Geometry check sheet. Reference: the model listing, model coordinates, mm. A direction names the side the tool comes from. Coordinates: 2 decimals unless noted, no trailing zeros. Loops run counter-clockwise (first coordinate to the right, second up) from the corner with the lowest first, then second, coordinate; pieces in that order, holes last.
from build123d import *

# Parameters (mm, degrees)
F0_W     = 33
F0_H     = 14
F1_DEPTH = 10
F2_W     = 33
F2_H     = 10.2
F3_DEPTH = 2
F4_D     = 3
F4_DEPTH = 20.5
F4_TIP   = 0.9012909285
F6_D     = 2.3
F6_DEPTH = 20.5
F6_TIP   = 0.6909897119


with BuildPart() as f1:
    # F0 (on Top) → F1 (new body)
    with BuildSketch(Plane.XY):
        Rectangle(F0_W, F0_H)
    extrude(amount=F1_DEPTH)

    # F2 (on face) → F3 (cut)
    with BuildSketch(Plane.XY.offset(10)):
        Rectangle(F2_W, F2_H)
    extrude(amount=-F3_DEPTH, mode=Mode.SUBTRACT)

    # F4
    with Locations(Plane(origin=(0, 0, 0), x_dir=(1, 0, 0), z_dir=(0, 0, -1))):
        with Locations((-12, 0)):
            Hole(F4_D / 2, depth=F4_DEPTH)
            with Locations((0, 0, -(F4_DEPTH + F4_TIP / 2))):  # 118° drill point
                Cone(0, F4_D / 2, F4_TIP, mode=Mode.SUBTRACT)

    # F6
    with Locations(Plane.YZ.offset(16.5)):
        with Locations((0, 4)):
            Hole(F6_D / 2, depth=F6_DEPTH)
            with Locations((0, 0, -(F6_DEPTH + F6_TIP / 2))):  # 118° drill point
                Cone(0, F6_D / 2, F6_TIP, mode=Mode.SUBTRACT)


solid = f1.part
1) Access from +Z, -Z, +X, -X, +Y, -Y to the whole of each face (thin tool, end or side, straight path). Record for faces 1 (the flat face through (0, 0, 8)), 2 (the cylindrical face through (6.11, 0.15, 5.14)), 3 (the flat face through (0, -6, 10)).
Data:
face 1: +Z, +X, -X
face 2: +X
face 3: +Z, +X, -X, +Y, -Y
2) Section check A-A on x = -12. Record the cut outline in (y, z).
Data:
outline: (-7, 0) - (-1.5, 0) - (-1.5, 8) - (-5.1, 8) - (-5.1, 10) - (-7, 10) - close; (1.5, 0) - (7, 0) - (7, 10) - (5.1, 10) - (5.1, 8) - (1.5, 8) - close
3) Section check D-D on x = -8. Record the cut outline in (y, z).
Data:
outline: (-7, 0) - (7, 0) - (7, 10) - (5.1, 10) - (5.1, 8) - (-5.1, 8) - (-5.1, 10) - (-7, 10) - close
4) Section check C-C on x = 2. Record the cut outline in (y, z).
Data:
outline: (-7, 0) - (7, 0) - (7, 10) - (5.1, 10) - (5.1, 8) - (-5.1, 8) - (-5.1, 10) - (-7, 10) - close; hole circle Ø2.3 at (0, 4)
5) Depth check by flat-ended pin: pin 1 (2 mm diameter, centred on y = 0, z = 4, fed in from +X); pin 2 (4 mm diameter, centred on x = -12.5, y = -3, fed in from +Z); pin 3 (2.5 mm diameter, centred on x = -12, y = 0, fed in from +Z). Enter the tip coordinate at first touch or a pass-through.
Data:
pin 1: stops at x = -4.09
pin 2: stops at z = 8
pin 3: passes through
6) Section check B-B on z = 8.75. Record the cut outline in (x, y).
Data:
outline: (-16.5, -7) - (16.5, -7) - (16.5, -5.1) - (-16.5, -5.1) - close; (-16.5, 5.1) - (16.5, 5.1) - (16.5, 7) - (-16.5, 7) - close
7) Mould release check, pull along Y, two halves, no side actions. Record for faces 4 (the flat face through (0, 7, 5)), 5 (the flat face through (0, -7, 5)), 6 (the cylindrical face through (-10.5, -0.07, 4.06)): +Y half, -Y half, draft (parallel to the pull), parting line (faces both ways), or undercut.
Data:
face 4: +Y half
face 5: -Y half
face 6: undercut
8) Material ranges on probe 1 along Y at (x, z) = (14.5, 9.5); probe 2 along Z at (x, y) = (11.75, 0); probe 3 along Z at (x, y) = (12, -4.5), recorded low to high.
Data:
probe 1: y = -7 to -5.1, 5.1 to 7
probe 2: z = 0 to 2.85, 5.15 to 8
probe 3: z = 0 to 8
